The listing builds one solid part. Answer for the finished solid, in the listing's coordinates (mm). Face numbers are marked on the shaded views. Coordinates: 2 decimals unless noted, no trailing zeros. Order: outer loops, then holes, each group sorted by start corner. A loop starts at its lowest first (then second) coordinate and runs counter-clockwise, first axis right, second up.
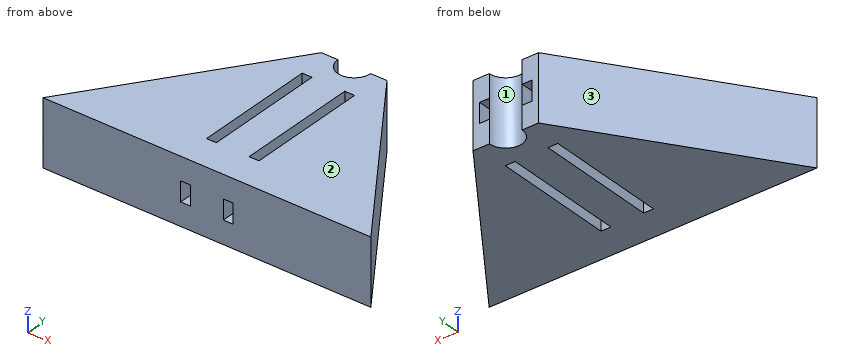
```python
from build123d import *

# Parameters (mm, degrees)
BOSS_EXTRUDE1_DEPTH = 10
SKETCH4_W           = 1.5
SKETCH4_H           = 3
CUT_EXTRUDE2_DEPTH  = 29.5
SKETCH5_W           = 1.5
SKETCH5_H           = 18.5
CUT_EXTRUDE3_DEPTH  = 11


with BuildPart() as part:
    # Sketch1 → Boss-Extrude1 (new body)
    with BuildSketch(Plane.XY):
        with BuildLine():
            Line((-25, -28.5), (25, -28.5))
            Line((25, -28.5), (5, 0))
            Line((5, 0), (2.5, 0))
            ThreePointArc((2.5, 0), (0, -2.5), (-2.5, 0))
            Line((-2.5, 0), (-5, 0))
            Line((-5, 0), (-25, -28.5))
        make_face()
    extrude(amount=BOSS_EXTRUDE1_DEPTH)

    # Sketch4 → Cut-Extrude2 (cut, through all)
    with BuildSketch(Plane.XZ.offset(28.5)):
        with Locations((-3.25, 5)):
            Rectangle(SKETCH4_W, SKETCH4_H)
    cut_extrude2 = extrude(amount=-CUT_EXTRUDE2_DEPTH, mode=Mode.SUBTRACT)

    # Mirror1: Cut-Extrude2 across plane
    add(cut_extrude2.mirror(Plane(origin=(0, 0, 0), x_dir=(0, 0, 1), z_dir=(1, 0, 0))), mode=Mode.SUBTRACT)

    # Sketch5 → Cut-Extrude3 (cut, through all)
    with BuildSketch(Plane.XY.offset(10)):
        with Locations((-3.25, -14.25)):
            Rectangle(SKETCH5_W, SKETCH5_H)
        with Locations((3.25, -14.25)):
            Rectangle(SKETCH5_W, SKETCH5_H)
    extrude(amount=-CUT_EXTRUDE3_DEPTH, mode=Mode.SUBTRACT)


solid = part.part
```
1) Straight lines are drawn through the part: probe 1 along Y at (x, z) = (-3, 6.75); probe 2 along X at (y, z) = (-20.5, 4); probe 3 along X at (y, z) = (-16.25, 5.75). For each, find the intervals that lie inside material, in ascending order.
2) The mould has two halves that part along X. Classify the marked faces 1, 2 and 3: released by +X, released by -X, zero draft, split by the parting line, or undercut.
3) A cutting plane is placed at A-A, the plane z = 4.75. Write down the section's boundary in (x, y), plus the area to 3 significant figures.
4) This flat-tipped pin is pushed along its axis until it touches: P1, Ø5, axis at y = -22.5, z = 7, coming from the +X side. Where does it stop, or does it pass through?
5) A cutting plane is placed at D-D, the plane y = -22.5. Write down the section's boundary in (x, z), plus the area to 3 significant figures.
6) A cutting plane is placed at C-C, the plane z = 7.5. Write down the section's boundary in (x, y).
7) A cutting plane is placed at B-B, the plane x = 3. Write down the section's boundary in (y, z).
Working result:
1. probe 1: y = -28.5 to -23.5, -5 to 0
1. probe 2: x = -19.39 to -4, -2.5 to 2.5, 4 to 19.39
1. probe 3: x = -16.4 to -4, -2.5 to 2.5, 4 to 16.4
2. face 1: undercut
2. face 2: zero draft
2. face 3: released by -X
3. outline: (-25, -28.5) - (-4, -28.5) - (-4, 0) - (-5, 0) - close; (-2.5, -28.5) - (2.5, -28.5) - (2.5, 0) arc R2.5 cw to (-2.5, 0) - close; (4, -28.5) - (25, -28.5) - (5, 0) - (4, 0) - close
3. area: 760 mm2
4. P1: stops at x = 22.54
5. outline: (-20.79, 0) - (-4, 0) - (-4, 10) - (-20.79, 10) - close; (-2.5, 0) - (2.5, 0) - (2.5, 10) - (-2.5, 10) - close; (4, 0) - (20.79, 0) - (20.79, 10) - (4, 10) - close
5. area: 386 mm2
6. outline: (-25, -28.5) - (25, -28.5) - (5, 0) - (2.5, 0) arc R2.5 cw to (-2.5, 0) - (-5, 0) - close; hole (-4, -23.5) - (-2.5, -23.5) - (-2.5, -5) - (-4, -5) - close; hole (2.5, -23.5) - (4, -23.5) - (4, -5) - (2.5, -5) - close
7. outline: (-28.5, 0) - (-23.5, 0) - (-23.5, 3.5) - (-28.5, 3.5) - close; (-28.5, 6.5) - (-23.5, 6.5) - (-23.5, 10) - (-28.5, 10) - close; (-5, 0) - (0, 0) - (0, 3.5) - (-5, 3.5) - close; (-5, 6.5) - (0, 6.5) - (0, 10) - (-5, 10) - close
